Could you check a few things on this model? Use its own coordinates, in mm. A direction names the side the tool comes from. Give positions to 0.01 mm unless a question says otherwise; leave off trailing zeros. Loops run counter-clockwise (first coordinate to the right, second up) from the corner with the lowest first, then second, coordinate; pieces in that order, holes last. Notation, with made-up numbers: M 84.5,25 L 106.5,25 A13 ccw 106.5,44 Z; hole C -39,48.5 d3. An arc over 180 degrees is marked long. Return JSON: item names as keys, results as strings. Group by question number.
1. If we section it at B-B (z = 30): Write out the boundary of the cut face in (x, y), plus the area to 3 significant figures.
2. For faces 1 (the flat face through (5, -15, 3)), 2 (the flat face through (-9, -10, 3)), which set-ups out of +Z, -Z, +X, -X, +Y, -Y let a thin tool reach every point of the face, with its end or its side?
3. If we section it at A-A (y = 0): Write out the boundary of the cut face in (x, z), plus the area to 3 significant figures.
4. Please list where these lines run through material, in increasing order: line 1 (X direction, y = 3, z = 2.5); line 2 (X direction, y = -4, z = 14); line 3 (Z direction, x = 20, y = 6).
5. For pin 1 (1.6 mm diameter, centred on x = -9, y = -13.5, fed in from +Z); pin 2 (8 mm diameter, centred on x = 17.5, z = 14, fed in from -Y); pin 3 (4 mm diameter, centred on y = 16.5, z = 3, fed in from -X); pin 4 (1.5 mm diameter, centred on y = 12.5, z = 2.5, fed in from -X), each with a flat end and sliding along its axis, tell me the tip position at first contact or that it passes through.
6. If we mould it in two halves opening along X, with no side actions, what happens to faces 3 (the flat face through (-2, -0.3, 14.5)), 4 (the flat face through (-4, 10, 3)), 5 (the flat face through (0, 0, 51))? For each: +X half, -X half, draft (parallel to the pull), parting line (faces both ways), or undercut.
7. If we section it at C-C (y = -17): Write out the boundary of the cut face in (x, z), plus the area to 3 significant figures.
8. If we section it at D-D (z = 5): State how many separate pieces and enclosed holes the cut face has, plus the area to 3 significant figures.
```python
from build123d import *

# Parameters (mm, degrees)
F0_R     = 4
F0_W     = 4
F0_H     = 50
F1_DEPTH = 20
F2_W     = 2
F2_H     = 10
F3_DEPTH = 5
F4_R     = 15
F5_DEPTH = 25
F6_DEPTH = 5


with BuildPart() as f1:
    # F0 (on Front) → F1 (new body, symmetric)
    with BuildSketch(Plane.XZ):
        with BuildLine():
            Line((-20, -1), (20, -1))
            ThreePointArc((20, -1), (22.236068, 8.472136), (16, 1))
            Line((16, 1), (2, 1))
            Line((2, 1), (-2, 1))
            Line((-2, 1), (-16, 1))
            Line((-16, 1), (-17.354249, 1))
            ThreePointArc((-17.354249, 1), (-18.585786, 0.258343), (-20, 0))
            Line((-20, 0), (-20, -1))
        make_face()
        with Locations((20, 4)):
            Circle(F0_R, mode=Mode.SUBTRACT)
        with BuildLine():
            ThreePointArc((-16, 1), (-22.236068, 8.472136), (-20, -1))
            Line((-20, -1), (-20, 0))
            ThreePointArc((-20, 0), (-22.828427, 6.828427), (-16, 4))
            ThreePointArc((-16, 4), (-16.354249, 2.354249), (-17.354249, 1))
            Line((-17.354249, 1), (-16, 1))
        make_face()
        with Locations((0, 26)):
            Rectangle(F0_W, F0_H)
    extrude(amount=F1_DEPTH, both=True)

    # F2 (on face) → F3 (join)
    with BuildSketch(Plane.XY.offset(1)):
        with Locations((8.5, -15)):
            Rectangle(F2_W, F2_H)
        with Locations((4, -15)):
            Rectangle(F2_W, F2_H)
        with Locations((-8.5, -15)):
            Rectangle(F2_W, F2_H)
        with Locations((-4, -15)):
            Rectangle(F2_W, F2_H)
        with Locations((8.5, 15)):
            Rectangle(F2_W, F2_H)
        with Locations((-8.5, 15)):
            Rectangle(F2_W, F2_H)
        with Locations((-4, 15)):
            Rectangle(F2_W, F2_H)
        with Locations((4, 15)):
            Rectangle(F2_W, F2_H)
    extrude(amount=F3_DEPTH)

    # F4 (on face) → F5 (cut)
    with BuildSketch(Plane.YZ.offset(2)):
        with Locations((0, 30)):
            Circle(F4_R)
    extrude(amount=-F5_DEPTH, mode=Mode.SUBTRACT)

    # F2 (on face) → F6 (join)
    with BuildSketch(Plane.XY.offset(1)):
        with Locations((8.5, -15)):
            Rectangle(F2_W, F2_H)
        with Locations((4, -15)):
            Rectangle(F2_W, F2_H)
        with Locations((-8.5, -15)):
            Rectangle(F2_W, F2_H)
        with Locations((-4, -15)):
            Rectangle(F2_W, F2_H)
        with Locations((8.5, 15)):
            Rectangle(F2_W, F2_H)
        with Locations((-8.5, 15)):
            Rectangle(F2_W, F2_H)
        with Locations((-4, 15)):
            Rectangle(F2_W, F2_H)
        with Locations((4, 15)):
            Rectangle(F2_W, F2_H)
    extrude(amount=F6_DEPTH)


solid = f1.part
```
Answer:
{
 "1": {"outline": "M -2,-20 L 2,-20 L 2,-15 L -2,-15 Z; M -2,15 L 2,15 L 2,20 L -2,20 Z", "area": "40.0 mm²"},
 "2": {"face 1": "+Z, +Y, -Y", "face 2": "+Z"},
 "3": {"outline": "M -20,-1 L 20,-1 A5 ccw long 16,1 L 2,1 L 2,15 L -2,15 L -2,1 L -16,1 A5 ccw long Z; M -2,45 L 2,45 L 2,51 L -2,51 Z; hole M -20,0 A4 ccw -17.35,1 A4 ccw -16,4 A4 ccw long Z; hole C 20,4 d8", "area": "205 mm²"},
 "4": {"line 1": "x = -24.77 to -23.71, -16.29 to -15.23, -2 to 2, 15.23 to 16.29, 23.71 to 24.77", "line 2": "x = -2 to 2", "line 3": "z = -1 to 0, 8 to 9"},
 "5": {"pin 1": "stops at z = 6", "pin 2": "passes through", "pin 3": "stops at x = -25", "pin 4": "stops at x = -24.94"},
 "6": {"face 3": "undercut", "face 4": "undercut", "face 5": "draft"},
 "7": {"outline": "M -20,-1 L 20,-1 A5 ccw long 16,1 L 9.5,1 L 9.5,6 L 7.5,6 L 7.5,1 L 5,1 L 5,6 L 3,6 L 3,1 L 2,1 L 2,51 L -2,51 L -2,1 L -3,1 L -3,6 L -5,6 L -5,1 L -7.5,1 L -7.5,6 L -9.5,6 L -9.5,1 L -16,1 A5 ccw long Z; hole M -20,0 A4 ccw -17.35,1 A4 ccw -16,4 A4 ccw long Z; hole C 20,4 d8", "area": "365 mm²"},
 "8": {"separate pieces": "13", "enclosed holes": "0", "area": "484 mm²"}
}
